```python
from build123d import *

# Parameters (mm, degrees)
BOSS_EXTRUDE1_DEPTH = 2.5
CUT_EXTRUDE1_DEPTH  = 3.5
BOSS_EXTRUDE2_DEPTH = 4.3
CUT_EXTRUDE2_DEPTH  = 20
SKETCH5_R           = 1.5
BOSS_EXTRUDE3_DEPTH = 1
SKETCH6_R           = 1.5
BOSS_EXTRUDE4_DEPTH = 1
FILLET1_R           = 0.9


with BuildPart() as part:
    # Sketch1 → Boss-Extrude1 (new body)
    with BuildSketch(Plane(origin=(0, 0, 0), x_dir=(1, 0, 0), z_dir=(0, 1, 0))):
        with BuildLine():
            Line((-6.212908396, -17), (6.212908396, -17))
            ThreePointArc((6.212908396, -17), (13.840534019, -13.840534019), (17, -6.212908396))
            Line((17, -6.212908396), (17, 6.212908396))
            ThreePointArc((17, 6.212908396), (13.840534019, 13.840534019), (6.212908396, 17))
            Line((6.212908396, 17), (-6.212908396, 17))
            ThreePointArc((-6.212908396, 17), (-13.840534019, 13.840534019), (-17, 6.212908396))
            Line((-17, 6.212908396), (-17, -6.212908396))
            ThreePointArc((-17, -6.212908396), (-13.840534019, -13.840534019), (-6.212908396, -17))
        make_face()
    extrude(amount=BOSS_EXTRUDE1_DEPTH)

    # Sketch2 → Cut-Extrude1 (cut, through all)
    with BuildSketch(Plane(origin=(0, 2.5, 0), x_dir=(1, 0, 0), z_dir=(0, 1, 0))):
        with BuildLine():
            Line((5.4, 3.7), (5.6, 3.7))
            ThreePointArc((5.6, 3.7), (6.589949494, 3.289949494), (7, 2.3))
            Line((7, 2.3), (7, -3.972202362))
            ThreePointArc((7, -3.972202362), (7.915239118, -5.353525898), (9.544072948, -5.049194321))
            ThreePointArc((9.544072948, -5.049194321), (10.621026492, -3.477336416), (11, -1.61))
            Line((11, -1.61), (11, 6.212908396))
            ThreePointArc((11, 6.212908396), (9.597893331, 9.597893331), (6.212908396, 11))
            Line((6.212908396, 11), (-6.212908396, 11))
            ThreePointArc((-6.212908396, 11), (-9.597893331, 9.597893331), (-11, 6.212908396))
            Line((-11, 6.212908396), (-11, -1.61))
            ThreePointArc((-11, -1.61), (-10.621026492, -3.477336416), (-9.544072948, -5.049194321))
            ThreePointArc((-9.544072948, -5.049194321), (-7.915239118, -5.353525898), (-7, -3.972202362))
            Line((-7, -3.972202362), (-7, 2.3))
            ThreePointArc((-7, 2.3), (-6.589949494, 3.289949494), (-5.6, 3.7))
            Line((-5.6, 3.7), (-5.4, 3.7))
            ThreePointArc((-5.4, 3.7), (-4.410050506, 3.289949494), (-4, 2.3))
            Line((-4, 2.3), (-4, -7.9))
            ThreePointArc((-4, -7.9), (-4.439339828, -8.960660172), (-5.5, -9.4))
            Line((-5.5, -9.4), (-6.21, -9.4))
            ThreePointArc((-6.21, -9.4), (-11.718361825, -7.118361825), (-14, -1.61))
            Line((-14, -1.61), (-14, 6.212908396))
            ThreePointArc((-14, 6.212908396), (-11.719213675, 11.719213675), (-6.212908396, 14))
            Line((-6.212908396, 14), (6.212908396, 14))
            ThreePointArc((6.212908396, 14), (11.719213675, 11.719213675), (14, 6.212908396))
            Line((14, 6.212908396), (14, -1.61))
            ThreePointArc((14, -1.61), (11.718361825, -7.118361825), (6.21, -9.4))
            Line((6.21, -9.4), (5.5, -9.4))
            ThreePointArc((5.5, -9.4), (4.439339828, -8.960660172), (4, -7.9))
            Line((4, -7.9), (4, 2.3))
            ThreePointArc((4, 2.3), (4.410050506, 3.289949494), (5.4, 3.7))
        make_face()
    extrude(amount=-CUT_EXTRUDE1_DEPTH, mode=Mode.SUBTRACT)

    # Sketch3 → Boss-Extrude2 (add)
    with BuildSketch(Plane(origin=(0, 2.5, 0), x_dir=(1, 0, 0), z_dir=(0, 1, 0))):
        with BuildLine():
            Line((-8.5, 8), (8.5, 8))
            ThreePointArc((8.5, 8), (10.621320344, 7.121320344), (11.5, 5))
            Line((11.5, 5), (11.5, 1))
            ThreePointArc((11.5, 1), (10.621320344, -1.121320344), (8.5, -2))
            Line((8.5, -2), (-8.5, -2))
            ThreePointArc((-8.5, -2), (-10.621320344, -1.121320344), (-11.5, 1))
            Line((-11.5, 1), (-11.5, 5))
            ThreePointArc((-11.5, 5), (-10.621320344, 7.121320344), (-8.5, 8))
        make_face()
    extrude(amount=BOSS_EXTRUDE2_DEPTH)

    # Sketch4 → Cut-Extrude2 (cut, through all)
    with BuildSketch(Plane.XY.offset(2)):
        Polygon((-11.5, 5), (-6.5, 5), (-3.15, 6.8), (3.15, 6.8), (6.5, 5), (11.5, 5), (14.66460311, 7.657087543), (13.998030241, 12.878575014), (-15.83110563, 15.267127793), (-17.386442324, 7.657087543), align=None)
        Polygon((3.15, 3.762686567), (-3.15, 3.762686567), (-5.5, 2.5), (5.5, 2.5), align=None)
    extrude(amount=-CUT_EXTRUDE2_DEPTH, mode=Mode.SUBTRACT)

    # Sketch5 → Boss-Extrude3 (add)
    with BuildSketch(Plane(origin=(0, 5, 0), x_dir=(1, 0, 0), z_dir=(0, 1, 0))):
        with Locations((9, 3)):
            Circle(SKETCH5_R)
    boss_extrude3 = extrude(amount=BOSS_EXTRUDE3_DEPTH)

    # Mirror1: Boss-Extrude3 across plane
    add(boss_extrude3.mirror(Plane(origin=(0, 0, 0), x_dir=(0, 0, 1), z_dir=(1, 0, 0))))

    # Sketch6 → Boss-Extrude4 (add)
    with BuildSketch(Plane(origin=(0, 6.8, 0), x_dir=(1, 0, 0), z_dir=(0, 1, 0))):
        with Locations((0, 3)):
            Circle(SKETCH6_R)
    extrude(amount=BOSS_EXTRUDE4_DEPTH)

    # Fillet1
    fillet1_edges = [part.edges().sort_by_distance(p)[0] for p in [
        (-1.5, 7.8, -3),
    ]]
    fillet(fillet1_edges, radius=FILLET1_R)


solid = part.part
```
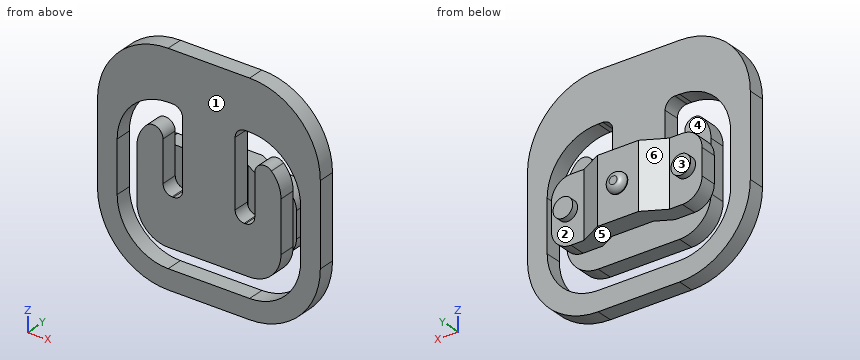
Build history of the part. All positions in model axes, mm. Face numbers are marked on the shaded views. A direction names the side the tool comes from. Coordinates: 2 decimals unless noted, no trailing zeros. Order: outer loops, then holes, each group sorted by start corner. A loop starts at its lowest first (then second) coordinate and runs counter-clockwise, first axis right, second up. Notation, with made-up numbers: (53.25, 26) -> (69.25, 26) arc R15 cw to (69.25, 50) -> close; hole circle Ø11 at (-21.75, 68.25). An arc over 180 degrees is marked (long way). Answer in a Markdown table with one row per item. Add a question column.
Q1. Mould opens along X. For the marked faces 1 and 2 say: +X half, -X half, draft (parallel to the pull), parting line (faces both ways), or undercut.
Q2. Band-saw the part on B-B, the plane z = -12. List the corners of the cut face in (x, y).
Q3. Band-saw the part on A-A, the plane x = 2. List the corners of the cut face in (y, z), then the cut area to 3 significant figures.
Q4. Which spindle directions (+Z, -Z, +X, -X, +Y, -Y) get a long thin tool onto all of the face, cutting with end or side? Do the marked faces 3, 4, 5 and 6. Say none if no direction does.
Q5. Band-saw the part on D-D, the plane z = 2.5. List the corners of the cut face in (x, y), then the cut area to 3 significant figures.
Q6. Band-saw the part on C-C, the plane y = 3.25. List the corners of the cut face in (x, z), then the cut area to 3 significant figures.
Q7. Drop flat-ended pins along their axis: pin 1 (0.9 mm diameter, centred on x = 8.5, z = -2.5, fed in from +Y); pin 2 (5 mm diameter, centred on x = 0.5, z = 10.5, fed in from +Y); pin 3 (1.5 mm diameter, centred on x = -9.5, z = -0.5, fed in from +Y). Give the stop position or say it passes through.
Q8. Wall check: line 1 along X through (y, z) = (1.5, -5.5); line 2 along Z through (x, y) = (-5, 2); line 3 along Y through (x, z) = (-11.5, -12.5). Give the ranges that are in metal, low to high. Write a range as [from, to].
Answers follow:
| question | item | result |
|---|---|---|
| 1 | face 1 | draft |
| 1 | face 2 | undercut |
| 2 | outline | (-15.32, 0) -> (-11.42, 0) -> (-11.42, 2.5) -> (-15.32, 2.5) -> close; (11.42, 0) -> (15.32, 0) -> (15.32, 2.5) -> (11.42, 2.5) -> close |
| 3 | outline | (0, -17) -> (2.5, -17) -> (2.5, -14) -> (0, -14) -> close; (0, -11) -> (2.5, -11) -> (2.5, 17) -> (0, 17) -> close; (3.76, -8) -> (6.8, -8) -> (6.8, 2) -> (3.76, 2) -> close |
| 3 | area | 108 mm^2 |
| 4 | face 3 | +Z, -Z, -X, +Y |
| 4 | face 4 | +Z, -X, +Y |
| 4 | face 5 | -Z, +X, -X, +Y |
| 4 | face 6 | +Z, -Z, +Y |
| 5 | outline | (-17, 0) -> (-13.95, 0) -> (-13.95, 2.5) -> (-17, 2.5) -> close; (-10.92, 0) -> (-7, 0) -> (-7, 2.5) -> (-10.92, 2.5) -> close; (-4, 0) -> (4, 0) -> (4, 2.5) -> (-4, 2.5) -> close; (7, 0) -> (10.92, 0) -> (10.92, 2.5) -> (7, 2.5) -> close; (13.95, 0) -> (17, 0) -> (17, 2.5) -> (13.95, 2.5) -> close |
| 5 | area | 54.8 mm^2 |
| 6 | outline | (-11.5, -5) arc R3 ccw to (-8.5, -8) -> (-4.1, -8) -> (-4.1, 2) -> (-8.5, 2) arc R3 ccw to (-11.5, -1) -> close; (4.1, -8) -> (8.5, -8) arc R3 ccw to (11.5, -5) -> (11.5, -1) arc R3 ccw to (8.5, 2) -> (4.1, 2) -> close |
| 6 | area | 140 mm^2 |
| 7 | pin 1 | y = 6 |
| 7 | pin 2 | y = 2.5 |
| 7 | pin 3 | y = 5 |
| 8 | line 1 | [-17, -14], [-11, 11], [14, 17] |
| 8 | line 2 | [-17, -14], [-11, -3.64], [9.31, 17] |
| 8 | line 3 | [0, 2.5] |
